Input: dimensioned drawing with shaded views. Units: mm. Origin: part minimum x, y, z. A direction names the side the tool comes from. Coordinates: 2 decimals unless noted, no trailing zeros. Order: outer loops, then holes, each group sorted by start corner. A loop starts at its lowest first (then second) coordinate and runs counter-clockwise, first axis right, second up. Notation, with made-up numbers: (13, 46.5) -> (63, 46.5) arc R5 ccw to (63, 50.5) -> close; hole circle Ø9 at (5.5, 74.25). An arc over 180 degrees is marked (long way). Answer in a Markdown table with one row per item. Add a question column.
1) Set-up query: the marked faces 1, 2 and 3. Return all of +Z, -Z, +X, -X, +Y, -Y with unobstructed straight access to the full face (end or side cutting, diameter ignored); none if empty.
2) Contact query for flat-ended pins moving along their axis: P1, Ø3, axis at y = 17, z = 30.5, coming from the -X side; P2, Ø5, axis at x = 6, y = 5, coming from the +Z side; P3, Ø12, axis at x = 38, z = 12.5, coming from the +Y side; P4, Ø1.5, axis at y = 17, z = 30.5, coming from the -X side. Output: stop coordinate, or through.
3) Pull-direction query (X, two-part tool) for the marked faces 4, 5 and 6; classes: +X half, -X half, draft (parallel to the pull), parting line (faces both ways), or undercut.
4) Ray query, line 1 (X direction, y = 3.5, z = 31.5); line 2 (Y direction, x = 36, z = 10) (1 decimal); line 3 (Y direction, x = 33.5, z = 50.5). Return the intervals inside material, ascending. Write a range as from..to.
5) Section query D-D on x = 29. Return the cut outline in (y, z).
6) Section query B-B on z = 10.2. Return the cut outline in (x, y), then the cut area to 3 significant figures.
7) Section query A-A on y = 3.5. Return the cut outline in (x, z).
8) Section query C-C on z = 21.5. Return the cut outline in (x, y).
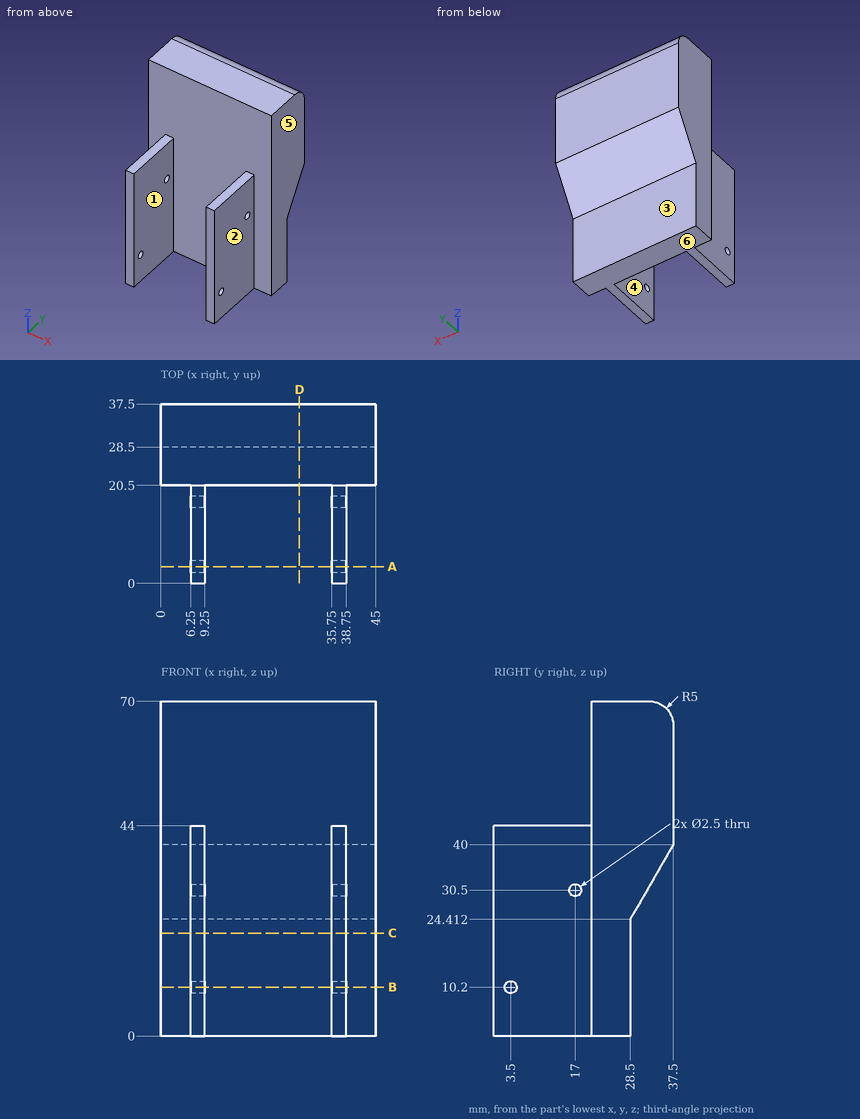
Result:
| question | item | result |
|---|---|---|
| 1 | face 1 | +Z, -Z, -Y |
| 1 | face 2 | +Z, -Z, +X, -Y |
| 1 | face 3 | -Z, +X, -X, +Y |
| 2 | P1 | x = 6.25 |
| 2 | P2 | z = 44 |
| 2 | P3 | y = 28.5 |
| 2 | P4 | through |
| 3 | face 4 | undercut |
| 3 | face 5 | +X half |
| 3 | face 6 | draft |
| 4 | line 1 | 6.25..9.25, 35.75..38.75 |
| 4 | line 2 | 0..2.3, 4.7..28.5 |
| 4 | line 3 | 20.5..37.5 |
| 5 | outline | (20.5, 0) -> (28.5, 0) -> (28.5, 24.41) -> (37.5, 40) -> (37.5, 65) arc R5 ccw to (32.5, 70) -> (20.5, 70) -> close |
| 6 | outline | (0, 20.5) -> (6.25, 20.5) -> (6.25, 4.75) -> (9.25, 4.75) -> (9.25, 20.5) -> (35.75, 20.5) -> (35.75, 4.75) -> (38.75, 4.75) -> (38.75, 20.5) -> (45, 20.5) -> (45, 28.5) -> (0, 28.5) -> close; (6.25, 0) -> (9.25, 0) -> (9.25, 2.25) -> (6.25, 2.25) -> close; (35.75, 0) -> (38.75, 0) -> (38.75, 2.25) -> (35.75, 2.25) -> close |
| 6 | area | 468 mm2 |
| 7 | outline | (6.25, 0) -> (9.25, 0) -> (9.25, 8.95) -> (6.25, 8.95) -> close; (6.25, 11.45) -> (9.25, 11.45) -> (9.25, 44) -> (6.25, 44) -> close; (35.75, 0) -> (38.75, 0) -> (38.75, 8.95) -> (35.75, 8.95) -> close; (35.75, 11.45) -> (38.75, 11.45) -> (38.75, 44) -> (35.75, 44) -> close |
| 8 | outline | (0, 20.5) -> (6.25, 20.5) -> (6.25, 0) -> (9.25, 0) -> (9.25, 20.5) -> (35.75, 20.5) -> (35.75, 0) -> (38.75, 0) -> (38.75, 20.5) -> (45, 20.5) -> (45, 28.5) -> (0, 28.5) -> close |
